Can you work these out from the model? Positions are in its coordinate system, mm. A direction names the side the tool comes from. Give positions to 0.01 mm unless a question says otherwise; leave off trailing zeros. Write each loop counter-clockwise with the first axis right and the second up, starting at its lowest first coordinate (ties: lowest second). Pieces come first, ordered by that corner, then holes. Notation, with made-up numbers: (32.25, 18) -> (89.25, 18) arc R11 ccw to (89.25, 29) -> close; hole circle Ø8 at (31.25, 3). An arc over 180 degrees is marked (long way). One line per item, written item: value.
from build123d import *

# Parameters (mm, degrees)
SKETCH4_W           = 290
SKETCH4_H           = 170
BOSS_EXTRUDE1_DEPTH = 45
SHELL1_T            = -5
SKETCH5_R           = 26.67
CUT_EXTRUDE1_DEPTH  = 40


with BuildPart() as part:
    # Sketch4 → Boss-Extrude1 (new body, symmetric)
    with BuildSketch(Plane(origin=(0, 0, 0), x_dir=(1, 0, 0), z_dir=(0, 1, 0))):
        with Locations((35, 0)):
            Rectangle(SKETCH4_W, SKETCH4_H)
    extrude(amount=BOSS_EXTRUDE1_DEPTH, both=True)

    # Shell1
    shell1_openings = [part.faces().sort_by_distance(p)[0] for p in [
        (35, 45, 0),
    ]]
    offset(amount=SHELL1_T, openings=shell1_openings, kind=Kind.INTERSECTION)

    # Sketch5 → Cut-Extrude1 (cut, symmetric)
    with BuildSketch(Plane.ZY.offset(110)):
        with Locations((-47.514984282, 0)):
            Circle(SKETCH5_R)
        with Locations((47.514984282, 0)):
            Circle(SKETCH5_R)
    extrude(amount=CUT_EXTRUDE1_DEPTH, both=True, mode=Mode.SUBTRACT)


solid = part.part
1) If we section it at D-D (z = 38): Write out the boundary of the cut face in (x, y), and give its area (3 significant figures).
Answer list:
outline: (-110, -45) -> (180, -45) -> (180, 45) -> (175, 45) -> (175, -40) -> (-105, -40) -> (-105, -24.91) -> (-110, -24.91) -> close; (-110, 24.91) -> (-105, 24.91) -> (-105, 45) -> (-110, 45) -> close
area: 2,050 mm^2
2) We'd pull the mould along Z, two halves only. Please class faces 4 (the face through (33, -40, -1)), 5 (the face through (33, 1, 85)), 6 (the face through (-110, 1, 1)): released by +Z, released by -Z, zero draft, split by the parting line, or undercut.
Answer list:
face 4: undercut
face 5: released by +Z
face 6: zero draft
3) Will this pin go through, and if not, where does the flat tip stop? pin 1 (1.5 mm diameter, centred on x = 37, z = 22, fed in from +Y).
Answer list:
pin 1: stops at y = -40
4) If we section it at A-A (x = 48): Write out the boundary of the cut face in (y, z).
Answer list:
outline: (-45, -85) -> (45, -85) -> (45, -80) -> (-40, -80) -> (-40, 80) -> (45, 80) -> (45, 85) -> (-45, 85) -> close
5) For faces 1 (the face through (33, -45, -1)), 2 (the face through (-107.535, 8.011, -22.077)), 3 (the face through (33, 3, -80)), which set-ups out of +Z, -Z, +X, -X, +Y, -Y let a thin tool reach every point of the face, with its end or its side?
Answer list:
face 1: +Z, -Z, +X, -X, -Y
face 2: -X
face 3: +Y
6) I need wall thicknesses on L1, parallel to Z at x = 48, y = 9; L2, parallel to X at y = -29, z = -57.5; L3, parallel to Y at x = -75, z = 8. Which ranges of each line are inside material? Lowest first, please.
Answer list:
L1: z = -85 to -80, 80 to 85
L2: x = -110 to -105, 175 to 180
L3: y = -45 to -40
7) If we section it at C-C (y = 0): Write out the boundary of the cut face in (x, z).
Answer list:
outline: (-110, -85) -> (180, -85) -> (180, 85) -> (-110, 85) -> (-110, 74.18) -> (-105, 74.18) -> (-105, 80) -> (175, 80) -> (175, -80) -> (-105, -80) -> (-105, -74.18) -> (-110, -74.18) -> close; (-110, -20.84) -> (-105, -20.84) -> (-105, 20.84) -> (-110, 20.84) -> close
8) If we section it at B-B (z = -34): Write out the boundary of the cut face in (x, y).
Answer list:
outline: (-110, -45) -> (180, -45) -> (180, 45) -> (175, 45) -> (175, -40) -> (-105, -40) -> (-105, -22.99) -> (-110, -22.99) -> close; (-110, 22.99) -> (-105, 22.99) -> (-105, 45) -> (-110, 45) -> close
